The listing builds one solid part. Answer for the finished solid, in the listing's coordinates (mm). Face numbers are marked on the shaded views. A direction names the side the tool comes from. Coordinates: 2 decimals unless noted, no trailing zeros. Order: outer loops, then holes, each group sorted by start corner. A loop starts at its lowest first (then second) coordinate and runs counter-clockwise, first axis right, second up. Notation, with made-up numbers: (15, -37) -> (71, -37) arc R33 cw to (71, -8) -> close; hole circle Ø5 at (50.5, 88). An arc over 180 degrees is marked (long way). Write item = value, one per line.
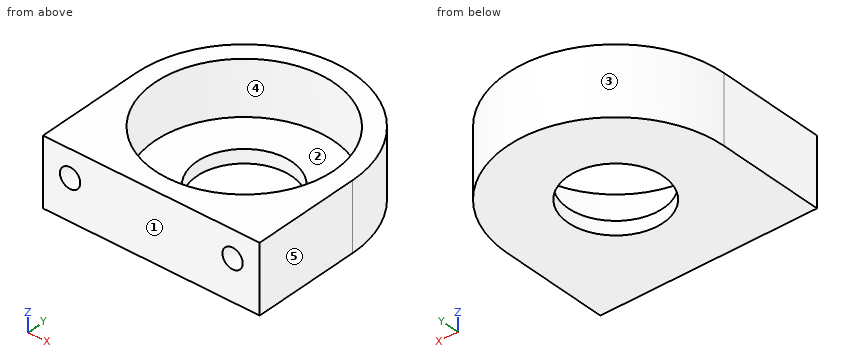
from build123d import *

# Parameters (mm, degrees)
F0_R     = 16
F1_DEPTH = 10
F2_W     = 32
F2_H     = 16
F3_DEPTH = 10
F4_R     = 13.2
F5_DEPTH = 8
F6_R     = 7
F7_DEPTH = 25
F8_R     = 1.5
F9_DEPTH = 7


with BuildPart() as f1:
    # F0 (on Top) → F1 (new body)
    with BuildSketch(Plane.XY):
        Circle(F0_R)
    extrude(amount=F1_DEPTH)

    # F2 (on face) → F3 (join)
    with BuildSketch(Plane.XY.offset(10)):
        with Locations((0, -8)):
            Rectangle(F2_W, F2_H)
    extrude(amount=-F3_DEPTH)

    # F4 (on face) → F5 (cut)
    with BuildSketch(Plane.XY.offset(10)):
        Circle(F4_R)
    extrude(amount=-F5_DEPTH, mode=Mode.SUBTRACT)

    # F6 (on face) → F7 (cut)
    with BuildSketch(Plane.XY.offset(2)):
        Circle(F6_R)
    extrude(amount=-F7_DEPTH, mode=Mode.SUBTRACT)

    # F8 (on face) → F9 (cut)
    with BuildSketch(Plane.XZ.offset(16)):
        with Locations((-12, 6)):
            Circle(F8_R)
        with Locations((12, 6)):
            Circle(F8_R)
    extrude(amount=-F9_DEPTH, mode=Mode.SUBTRACT)


solid = f1.part
Q1. Each of these flat-tipped pins is pushed along its axis until it touches: pin 1 Ø13 at (x, y) = (4.5, 1.5) entering from +Z; pin 2 Ø0.9 at (x, z) = (-12.5, 5.5) entering from -Y; pin 3 Ø3.5 at (x, z) = (12, 6) entering from +Y; pin 4 Ø11 at (x, y) = (0, 0) entering from +Z. Where does it stop, or does it pass through?
The answers:
pin_1 = 2
pin_2 = -9
pin_3 = 12.29
pin_4 = through
Q2. Section C-C, the plane y = 12 is taken. Give the vertices of the cut face in (x, z).
The answers:
outline = (-10.58, 0) -> (10.58, 0) -> (10.58, 10) -> (5.5, 10) -> (5.5, 2) -> (-5.5, 2) -> (-5.5, 10) -> (-10.58, 10) -> close
Q3. Find the intervals of material crossed by line 1 along Z through (x, y) = (12, -12.5); line 2 along Y through (x, z) = (0, 4.5); line 3 along Y through (x, z) = (0, 1.5), in increasing order.
The answers:
line_1 = 0 to 4.5, 7.5 to 10
line_2 = -16 to -13.2, 13.2 to 16
line_3 = -16 to -7, 7 to 16
Q4. A tool of negligible diameter and unlimited length cuts with its end or side. For the marked faces 4 and 5, from which of +Z, -Z, +X, -X, +Y, -Y can it reach the whole face along a straight path? Write none if from no direction.
The answers:
face_4 = +Z
face_5 = +Z, -Z, +X, +Y, -Y
Q5. Section B-B, the plane z = 8.75 is taken. Give the vertices of the cut face in (x, y).
The answers:
outline = (-16, -16) -> (16, -16) -> (16, 0) arc R16 ccw to (-16, 0) -> close; hole circle Ø26.4 at (0, 0)
Q6. The mould has two halves that part along X. Classify the marked faces 1, 2 and 3: released by +X, released by -X, zero draft, split by the parting line, or undercut.
The answers:
face_1 = zero draft
face_2 = undercut
face_3 = split by the parting line
Q7. Section A-A, the plane x = 0 is taken. Give the vertices of the cut face in (y, z), plus the area to 3 significant figures.
The answers:
outline = (-16, 0) -> (-7, 0) -> (-7, 2) -> (-13.2, 2) -> (-13.2, 10) -> (-16, 10) -> close; (7, 0) -> (16, 0) -> (16, 10) -> (13.2, 10) -> (13.2, 2) -> (7, 2) -> close
area = 80.8 mm2
Q8. Section D-D, the plane x = -12 is taken. Give the vertices of the cut face in (y, z).
The answers:
outline = (-16, 0) -> (10.58, 0) -> (10.58, 10) -> (5.5, 10) -> (5.5, 2) -> (-5.5, 2) -> (-5.5, 10) -> (-16, 10) -> (-16, 7.5) -> (-9, 7.5) -> (-9, 4.5) -> (-16, 4.5) -> close
